Check sheet for the modelled part. Datum: model origin and axes. Units: mm. A direction names the side the tool comes from. Give positions to 0.01 mm unless a question says otherwise; leave off trailing zeros. Order: outer loops, then holes, each group sorted by start corner. A loop starts at its lowest first (then second) coordinate and runs counter-clockwise, first axis right, second up. Notation, with made-up numbers: (50.25, 74) -> (87.25, 74) arc R29 ccw to (87.25, 111) -> close; hole circle Ø10 at (86, 38.25). An arc over 180 degrees is marked (long way). One line per question, with ' | ' between items.
```python
from build123d import *

# Parameters (mm, degrees)
SKETCH1_R                 = 70
BOSS_EXTRUDE1_DEPTH       = 2
SKETCH1_4_R               = 75
SKETCH1_4_R_2             = 70
BOSS_EXTRUDE2_DEPTH       = 100
M3_CLEARANCE_HOLE1_D      = 3.6
M3_CLEARANCE_HOLE1_DEPTH  = 2
M3_CLEARANCE_HOLE1_TIP    = 1.081549114
M10_CLEARANCE_HOLE1_D     = 12
M10_CLEARANCE_HOLE1_DEPTH = 2
M10_CLEARANCE_HOLE1_TIP   = 3.605163714


with BuildPart() as part:
    # Sketch1 → Boss-Extrude1 (new body)
    with BuildSketch(Plane(origin=(0, 0, 0), x_dir=(0, 0, -1), z_dir=(1, 0, 0))):
        Circle(SKETCH1_R)
    extrude(amount=BOSS_EXTRUDE1_DEPTH)

    # Sketch1<4> → Boss-Extrude2 (add)
    with BuildSketch(Plane(origin=(0, 0, 0), x_dir=(0, 0, -1), z_dir=(1, 0, 0))):
        Circle(SKETCH1_4_R)
        Circle(SKETCH1_4_R_2, mode=Mode.SUBTRACT)
    extrude(amount=BOSS_EXTRUDE2_DEPTH)

    # M3 Clearance Hole1
    with Locations(Plane(origin=(2, 0, 0), x_dir=(0, 0, -1), z_dir=(1, 0, 0))):
        with Locations((12.990381057, -7.5), (0, 15), (-12.990381057, -7.5)):
            Hole(M3_CLEARANCE_HOLE1_D / 2, depth=M3_CLEARANCE_HOLE1_DEPTH)
            with Locations((0, 0, -(M3_CLEARANCE_HOLE1_DEPTH + M3_CLEARANCE_HOLE1_TIP / 2))):  # 118° drill point
                Cone(0, M3_CLEARANCE_HOLE1_D / 2, M3_CLEARANCE_HOLE1_TIP, mode=Mode.SUBTRACT)

    # M10 Clearance Hole1
    with Locations(Plane(origin=(2, 0, 0), x_dir=(0, 0, -1), z_dir=(1, 0, 0))):
        with Locations((0, 0)):
            Hole(M10_CLEARANCE_HOLE1_D / 2, depth=M10_CLEARANCE_HOLE1_DEPTH)
            with Locations((0, 0, -(M10_CLEARANCE_HOLE1_DEPTH + M10_CLEARANCE_HOLE1_TIP / 2))):  # 118° drill point
                Cone(0, M10_CLEARANCE_HOLE1_D / 2, M10_CLEARANCE_HOLE1_TIP, mode=Mode.SUBTRACT)


solid = part.part
```
Q1. Section check B-B (x = 16). Enter the section's corners in (y, z).
Result sheet:
outline: circle Ø150 at (0, 0); hole circle Ø140 at (0, 0)
Q2. Depth check by flat-ended pin: pin 1 Ø10 at (x, y) = (81.5, -16) entering from +Z; pin 2 Ø8 at (x, z) = (66, -31.5) entering from +Y; pin 3 Ø3 at (y, z) = (15, 0) entering from +X; pin 4 Ø5 at (x, z) = (56, -50) entering from -Y. Enter the tip coordinate at first touch or a pass-through.
Result sheet:
pin 1: stops at z = 74.19 | pin 2: stops at y = 69.78 | pin 3: passes through | pin 4: stops at y = -58.04
Q3. Section check A-A (y = 0). Enter the section's corners in (x, z).
Result sheet:
outline: (0, -75) -> (100, -75) -> (100, -70) -> (2, -70) -> (2, -6) -> (0, -6) -> close; (0, 6) -> (2, 6) -> (2, 70) -> (100, 70) -> (100, 75) -> (0, 75) -> close
Q4. Mould release check, pull along Y, two halves, no side actions. Record for faces 3 (the face through (0, 1, -16)), 4 (the face through (2, -15, 1)), 5 (the face through (49.3, 74.362, 9.764)), 6 (the face through (1, 0, -6)): pulls with the +Y half, pulls with the -Y half, needs draft (parallel to the pull), parting line crosses it, or undercut.
Result sheet:
face 3: needs draft | face 4: undercut | face 5: parting line crosses it | face 6: undercut
Q5. Access from +Z, -Z, +X, -X, +Y, -Y to the whole of each face (thin tool, end or side, straight path). Record for faces 1 (the face through (50.314, -42.594, 55.55)), 2 (the face through (0.986, 16.785, -0.234)).
Result sheet:
face 1: +X | face 2: +X, -X
Q6. Section check D-D (y = -36). Enter the section's corners in (x, z).
Result sheet:
outline: (0, -65.8) -> (100, -65.8) -> (100, -60.03) -> (2, -60.03) -> (2, 60.03) -> (100, 60.03) -> (100, 65.8) -> (0, 65.8) -> close
Q7. Thickness scan on line 1 (Y direction, x = 1.45, z = 0); line 2 (Y direction, x = 91, z = -1); line 3 (Z direction, x = 0.9, y = -7.5). Record the ranges inside material, lowest first.
Result sheet:
line 1: y = -75 to -6, 6 to 13.2, 16.8 to 75 | line 2: y = -74.99 to -69.99, 69.99 to 74.99 | line 3: z = -74.62 to -14.79, -11.19 to 11.19, 14.79 to 74.62
Q8. Section check C-C (z = 62). Enter the section's corners in (x, y), and give its area (3 significant figures).
Result sheet:
outline: (0, -42.2) -> (100, -42.2) -> (100, -32.5) -> (2, -32.5) -> (2, 32.5) -> (100, 32.5) -> (100, 42.2) -> (0, 42.2) -> close | area: 2,070 mm2
